Autodesk Inventor part; units mm, degrees
ref_plane "YZ Plane" through (0, 0, 0) normal (1, 0, 0) x (0, 1, 0)
ref_plane "XZ Plane" through (0, 0, 0) normal (0, 1, 0) x (-1, 0, 0)
ref_plane "XY Plane" through (0, 0, 0) normal (0, 0, 1) x (1, 0, 0)
sketch "Boceto4" plane through (0, 0, 0) normal (0, 1, 0) x (-1, 0, 0)
  line L0 (0, 0) -> (165, 0)
  line L1 (165, 0) -> (165, -165)
  line L2 (165, -165) -> (0, -165)
  line L3 (0, -165) -> (0, 0)
  dimension "d6" = 165
  dimension "d7" = 165
extrude "Extrusión2" add sketch "Boceto4" along normal blind 6
sketch "Boceto5" plane through (0, 6, 0) normal (0, 1, 0) x (1, 0, 0)
  line L0 (-165, 0) -> (0, 0)
  line L1 (0, 165) -> (-165, 165)
  line L2 (0, 0) -> (-165, 165)
  line L3 (-165, 165) -> (0, 165)
  line L4 (-165, 165) -> (-165, 0)
  line L5 (0, 165) -> (-165, 0)
  circle A0 centre (-82.5, 82.5) radius 12
  circle A1 centre (-82.5, 82.5) radius 22.5
  line L6 (-82.5, 82.5) -> (-89.5711, 75.4289)
  line L7 (-82.5, 82.5) -> (-75.4289, 89.5711)
  line L8 (0, 0) -> (0, 165)
  line L9 (-82.5, 82.5) -> (-86.7426, 78.2574)
  line L10 (-86.7426, 78.2574) -> (-8.4853, 0)
  line L11 (-82.5, 82.5) -> (-78.2574, 86.7426)
  line L12 (-78.2574, 86.7426) -> (0, 8.4853)
  line L13 (-86.7426, 78.2574) -> (-165, 156.5147)
  line L14 (-78.2574, 86.7426) -> (-156.5147, 165)
  dimension "d10" = 24
  dimension "d11" = 45
  dimension "d14" = 6
  dimension "d15" = 6
extrude "Extrusión3" cut sketch "Boceto5" against normal through all contours A0 L13 L5 | L5 L10 A0 | L10 L5 L2 A0 | A0 L2 L5 L13 | L2 L5 L12 A0 | A0 L14 L5 L2 | L12 L5 A0 | A0 L5 L14
sketch "Boceto6" plane through (0, 6, 0) normal (0, 1, 0) x (1, 0, 0)
  line L0 (-165, 165) -> (-165, 0)
  line L1 (-165, 165) -> (0, 0)
  line L2 (0, 0) -> (0, 165)
  line L3 (-165, 0) -> (0, 165)
  circle A0 centre (-82.5, 82.5) radius 22.5
  line L4 (-82.5, 82.5) -> (-86.7426, 86.7426)
  line L5 (-86.7426, 86.7426) -> (-165, 8.4853)
  line L6 (-82.5, 82.5) -> (-78.2574, 78.2574)
  line L7 (-78.2574, 78.2574) -> (-156.5147, 0)
  line L8 (-165, 0) -> (0, 0)
  line L9 (-86.7426, 86.7426) -> (-8.4853, 165)
  line L10 (0, 165) -> (-165, 165)
  line L11 (-78.2574, 78.2574) -> (0, 156.5147)
  line L12 (-82.5, 82.5) -> (-78.2574, 86.7426)
  line L13 (-82.5, 82.5) -> (-78.2574, 86.7426)
  line L14 (-78.2574, 86.7426) -> (-156.5147, 165)
  line L15 (-82.5, 82.5) -> (-86.7426, 78.2574)
  line L16 (-86.7426, 78.2574) -> (-165, 156.5147)
  line L17 (-86.7426, 78.2574) -> (-8.4853, 0)
  line L18 (-165, 0) -> (-165, 165)
  line L19 (0, 165) -> (-165, 165)
  line L20 (0, 0) -> (0, 165)
  line L21 (-165, 0) -> (0, 0)
  line L22 (-165, 0) -> (0, 0)
  circle A1 centre (-82.5, 82.5) radius 12
  line L23 (0, 165) -> (-165, 165)
  line L24 (-165, 165) -> (-165, 0)
  line L25 (-165, 0) -> (0, 0)
  line L26 (0, 0) -> (0, 165)
  circle A2 centre (-82.5, 82.5) radius 12
  line L27 (0, 165) -> (-165, 165)
  line L28 (-165, 165) -> (-165, 0)
  line L29 (-165, 0) -> (0, 0)
  line L30 (0, 0) -> (0, 165)
  line L31 (0, -1.5147) -> (0, 8.4853)
  line L32 (0, 8.4853) -> (-165, 8.4853)
  line L33 (-156.5147, 0) -> (-156.5147, 165)
  line L34 (-8.4853, 0) -> (-8.4853, 165)
  line L35 (0, 156.5147) -> (-165, 156.5147)
  line L36 (-78.2574, 86.7426) -> (0, 8.4853)
  point P0 (-16.9706, 156.5147)
  point P1 (-148.0294, 156.5147)
  point P2 (-93.5911, 102.0764)
  point P3 (-71.4089, 102.0764)
  point P4 (-62.9236, 71.4089)
  point P5 (-8.4853, 16.9706)
  point P6 (-8.4853, 148.0294)
  point P7 (-62.9236, 93.5911)
  point P8 (-148.0294, 8.4853)
  point P9 (-16.9706, 8.4853)
  point P10 (-71.4089, 62.9236)
  point P11 (-93.5911, 62.9236)
  point P12 (-156.5147, 148.0294)
  point P13 (-156.5147, 16.9706)
  point P14 (-102.0764, 71.4089)
  point P15 (-102.0764, 93.5911)
  dimension "d18" = 45
  dimension "d19" = 6
  dimension "d20" = 6
  dimension "d21" = 6
  dimension "d22" = 6
  dimension "d24" = 10
extrude "Extrusión4" cut sketch "Boceto6" against normal through all contours L16 A0 L5 L33 | L35 L9 A0 L14 | L7 A0 L17 L32 | L34 L36 A0 L11
sketch "Boceto7" plane through (0, 6, 0) normal (0, 1, 0) x (1, 0, 0)
  point P0 (0, 0)
sketch "Boceto8" plane through (0, 6, 0) normal (0, 1, 0) x (1, 0, 0)
  line L0 (-148.0294, 156.5147) -> (-16.9706, 156.5147)
  line L1 (-165, 165) -> (-165, 0)
  line L2 (-16.9706, 8.4853) -> (-148.0294, 8.4853)
  line L3 (-16.9706, 156.5147) -> (-71.4089, 102.0764)
  circle A0 centre (-156.5147, 8.4853) radius 6.36
  point P0 (0, 0)
extrude "Extrusión5" cut sketch "Boceto8" against normal through all
CAD build for the part. Positions are in the model's coordinates, mm. A direction names the side the tool comes from. Round coordinates to 2 decimals unless told otherwise and drop trailing zeros. Write each loop counter-clockwise with the first axis right and the second up, starting at its lowest first coordinate (ties: lowest second). Pieces come first, ordered by that corner, then holes.
(1) Mould opens along Z. For faces 3 (the face through (-84, 3, -165)), 4 (the face through (-81, 3, 0)), 5 (the face through (-82.7, 3, -60)), 6 (the face through (-105, 3, -82.7)) say: pulls with the +Z half, pulls with the -Z half, needs draft (parallel to the pull), parting line crosses it, or undercut.
(2) Slice it at D-D, the plane x = -14.5. Write the cut outline in (y, z).
(3) Slice it at A-A, the plane x = -82.5. Write the cut outline in (y, z).
(4) Slice it at C-C, the plane y = 1.75. Write the cut outline in (x, z), and give its area (3 significant figures).
(5) Slice it at B-B, the plane z = -82.5. Write the cut outline in (x, y), and give its area (3 significant figures).
(6) Probe line 1 along Z through (x, y) = (-82.5, 2.1); line 2 along Z through (x, y) = (-37, 2.75); line 3 along X through (y, z) = (4.4, -116). List the from-to ranges inside material, lowest first.
(7) 3-axis set-ups, long thin cutter, end or side, ignore diameter. For faces 1 (the face through (-120.429, 3.042, -36.086)), 2 (the face through (-165, 3, -81)): which of +Z, -Z, +X, -X, +Y, -Y reach the whole face in a straight line?
From the geometry:
1. face 3: pulls with the -Z half
1. face 4: pulls with the +Z half
1. face 5: undercut
1. face 6: undercut
2. outline: (0, -165) - (6, -165) - (6, -142.01) - (0, -142.01) - close; (0, -22.99) - (6, -22.99) - (6, 0) - (0, 0) - close
3. outline: (0, -165) - (6, -165) - (6, -156.51) - (0, -156.51) - close; (0, -105) - (6, -105) - (6, -94.5) - (0, -94.5) - close; (0, -70.5) - (6, -70.5) - (6, -60) - (0, -60) - close; (0, -8.49) - (6, -8.49) - (6, 0) - (0, 0) - close
4. outline: (-165, -165) - (0, -165) - (0, 0) - (-165, 0) - close; hole circle Ø12.72 at (-156.51, -8.49); hole (-156.51, -148.03) - (-102.08, -93.59) arc R22.5 cw to (-102.08, -71.41) - (-156.51, -16.97) - close; hole (-148.03, -156.51) - (-16.97, -156.51) - (-71.41, -102.08) arc R22.5 cw to (-93.59, -102.08) - close; hole (-148.03, -8.49) - (-93.59, -62.92) arc R22.5 cw to (-71.41, -62.92) - (-16.97, -8.49) - close; hole circle Ø24 at (-82.5, -82.5); hole (-62.92, -93.59) - (-8.49, -148.03) - (-8.49, -16.97) - (-62.92, -71.41) arc R22.5 cw to start
4. area: 10,100 mm2
5. outline: (-165, 0) - (-156.51, 0) - (-156.51, 6) - (-165, 6) - close; (-105, 0) - (-94.5, 0) - (-94.5, 6) - (-105, 6) - close; (-70.5, 0) - (-60, 0) - (-60, 6) - (-70.5, 6) - close; (-8.49, 0) - (0, 0) - (0, 6) - (-8.49, 6) - close
5. area: 228 mm2
6. line 1: z = -165 to -156.51, -105 to -94.5, -70.5 to -60, -8.49 to 0
6. line 2: z = -165 to -156.51, -136.49 to -119.51, -45.49 to -28.51, -8.49 to 0
6. line 3: x = -165 to -156.51, -124.49 to -107.51, -57.49 to -40.51, -8.49 to 0
7. face 1: +Y, -Y
7. face 2: +Z, -Z, -X, +Y, -Y
